Input: part model. Units: mm. Frame: model coordinates. A direction names the side the tool comes from. Coordinates: 2 decimals unless noted, no trailing zeros. Order: outer loops, then holes, each group sorted by start corner. A loop starts at its lowest first (then second) coordinate and runs counter-clockwise, first axis right, second up. Notation, with made-up numbers: (59, 33) - (110, 33) arc R25 ccw to (110, 54) - close; hole circle Ø3 at (-7.75, 32.5). An arc over 180 degrees is marked (long way). Use a Markdown table: item, result. Add a question column.
Autodesk Inventor part; units mm, degrees
ref_plane "YZ Plane" through (0, 0, 0) normal (1, 0, 0) x (0, 1, 0)
ref_plane "XZ Plane" through (0, 0, 0) normal (0, 1, 0) x (-1, 0, 0)
ref_plane "XY Plane" through (0, 0, 0) normal (0, 0, 1) x (1, 0, 0)
sketch "Sketch1" plane through (0, 0, 0) normal (0, 1, 0) x (-1, 0, 0)
  circle A0 centre (0, 0) radius 17.78
  dimension "d0" = 35.56
extrude "Extrusion1" add sketch "Sketch1" along normal blind 10.16
sketch "Sketch2" plane through (0, 10.16, 0) normal (0, 1, 0) x (1, 0, 0)
  circle A0 centre (0, 0) radius 17.78
hole "Hole1" at (0, 10.16, 0) direction (0, -1, 0) diameter 6.35 end through all
sketch "Sketch3" plane through (0, 10.16, 0) normal (0, 1, 0) x (1, 0, 0)
  line L0 (0, 0) -> (-13.6144, 0)
  dimension "d10" = 13.6144
hole "Hole2" at (-13.6144, 10.16, 0) direction (0, -1, 0) diameter 4.9022 end through all
pattern_circular "Circular Pattern1" count 3 over 360 about axis through (0, -41.1455, 0) along (0, 1, 0) of "Hole2"
sketch "Sketch5" plane through (0, 10.16, 0) normal (0, 1, 0) x (1, 0, 0)
  circle A0 centre (-13.6144, 0) radius 2.4511
  circle A1 centre (6.8072, 11.7904) radius 2.4511
  line L0 (-13.6144, 0) -> (6.8072, 11.7904)
  circle A2 centre (6.8072, -11.7904) radius 2.4511
  line L1 (6.8072, 11.7904) -> (6.8072, -11.7904)
  line L2 (6.8072, -11.7904) -> (-13.6144, 0)
  line L3 (-13.6144, 0) -> (-13.6144, -11.7904)
  line L4 (-13.6144, -11.7904) -> (6.8072, -11.7904)
  line L5 (-13.6144, 0) -> (-13.6144, 11.7904)
  line L6 (-13.6144, 11.7904) -> (6.8072, 11.7904)
  circle A3 centre (-3.4036, 11.7904) radius 0.635
  circle A4 centre (-3.4036, -11.7904) radius 0.635
  point P0 (0, 0)
  dimension "d28" = 1.27
hole "Hole4" at (-3.4036, 10.16, 11.7904) at (-3.4036, 10.16, -11.7904) direction (0, -1, 0) diameter 1.905 end through all
sketch "Sketch15" plane through (0, 10.16, 0) normal (0, 1, 0) x (1, 0, 0)
  circle A0 centre (10.6172, -4.7625) radius 3.175
  circle A1 centre (10.6172, 4.7625) radius 3.175
  point P0 (0, 0)
shell "Shell3" thickness 0.635 removed faces 0
hole "Hole7" at (10.6172, 10.16, 4.7625) at (10.6172, 10.16, -4.7625) direction (0, -1, 0) diameter 6.35 depth 5.08
sketch "Sketch16" plane through (0, 10.16, 0) normal (0, 1, 0) x (1, 0, 0)
  circle A0 centre (10.6172, 4.7625) radius 3.175
  circle A1 centre (10.6172, 4.7625) radius 3.81
  circle A2 centre (10.6172, -4.7625) radius 3.175
  circle A3 centre (10.6172, -4.7625) radius 3.81
  circle A4 centre (10.6172, 4.7625) radius 3.175
  circle A5 centre (10.6172, -4.7625) radius 3.175
  point P0 (0, 0)
  dimension "d85" = 7.62
  dimension "d86" = 7.62
extrude "Extrusion7" add sketch "Sketch16" against normal blind 2.54 contours A3
extrude "Extrusion8" add sketch "Sketch16" against normal blind 7.62 contours A1
properties part number "water"
1) Contact query for flat-ended pins moving along their axis: P1, Ø5, axis at y = 5, z = 14, coming from the +X side; P2, Ø3, axis at y = 1.5, z = 6.5, coming from the -X side; P3, Ø5, axis at x = 10.62, z = 4.76, coming from the +Y side (3 decimals); P4, Ø5.5, axis at x = 0, z = 0, coming from the -Y side. Output: stop coordinate, or through.
2) Cut plane B-B (x = 0). Return the cut outline in (y, z) (3 decimals), and give its area (3 significant figures).
3) Material intervals for L1, parallel to Z at x = 0, y = 6 (3 decimals); L2, parallel to Z at x = 13, y = 3; L3, parallel to Y at x = -7, z = 1 (3 decimals), sorted ascending.
4) Reachability of faces 1 (the cylindrical face through (-3.69, 5.01, -10.88)), 2 (the cylindrical face through (-9.217, 5.018, -14.457)) from +Z, -Z, +X, -X, +Y, -Y: full face, straight path, thin tool, end or side. Return the list, or none.
5) Cut plane C-C (y = 8.5). State how many separate pieces and enclosed holes the cut face has, and give its area (3 significant figures).
6) Pull-direction query (X, two-part tool) for faces 3 (the flat face through (-4, 10.16, 0)), 4 (the cylindrical face through (3.85, 5.01, 17.36)), 5 (the flat face through (4, 0.635, 0)); classes: pulls with the +X half, pulls with the -X half, needs draft (parallel to the pull), parting line crosses it, or undercut.
7) Cut plane A-A (z = 0). Return the cut outline in (x, y) (1 decimal).
Computed:
| question | item | result |
|---|---|---|
| 1 | P1 | stops at x = 13.56 |
| 1 | P2 | stops at x = -17.06 |
| 1 | P3 | stops at y = 0.635 |
| 1 | P4 | passes through |
| 2 | outline | (0, -17.78) - (10.16, -17.78) - (10.16, -3.175) - (0, -3.175) - close; (0, 3.175) - (10.16, 3.175) - (10.16, 17.78) - (0, 17.78) - close; hole (0.635, -17.145) - (9.525, -17.145) - (9.525, -3.81) - (0.635, -3.81) - close; hole (0.635, 3.81) - (9.525, 3.81) - (9.525, 17.145) - (0.635, 17.145) - close |
| 2 | area | 59.7 mm2 |
| 3 | L1 | z = -17.78 to -17.145, -3.81 to -3.175, 3.175 to 3.81, 17.145 to 17.78 |
| 3 | L2 | z = -12.13 to -11.18, -7.74 to -6.86, -2.66 to -1.79, 11.18 to 12.13 |
| 3 | L3 | y = 0 to 0.635, 9.525 to 10.16 |
| 4 | face 1 | +Y, -Y |
| 4 | face 2 | none |
| 5 | separate pieces | 9 |
| 5 | enclosed holes | 9 |
| 5 | area | 155 mm2 |
| 6 | face 3 | needs draft |
| 6 | face 4 | parting line crosses it |
| 6 | face 5 | undercut |
| 7 | outline | (-17.8, 0) - (-16.1, 0) - (-16.1, 10.2) - (-17.8, 10.2) - close; (-11.2, 0) - (-3.2, 0) - (-3.2, 10.2) - (-11.2, 10.2) - close; (3.2, 0) - (17.8, 0) - (17.8, 10.2) - (3.2, 10.2) - close; hole (-17.1, 0.6) - (-16.7, 0.6) - (-16.7, 9.5) - (-17.1, 9.5) - close; hole (-10.5, 0.6) - (-3.8, 0.6) - (-3.8, 9.5) - (-10.5, 9.5) - close; hole (3.8, 0.6) - (17.1, 0.6) - (17.1, 9.5) - (3.8, 9.5) - close |
